Verification items for the finished model (mm, model axes). Coordinates: 2 decimals unless noted, no trailing zeros. Order: outer loops, then holes, each group sorted by start corner. A loop starts at its lowest first (then second) coordinate and runs counter-clockwise, first axis right, second up. Notation, with made-up numbers: M -21.5,-6 L -1.5,-6 A27 cw -1.5,22 Z; hole C -1.5,22 d5. An arc over 180 degrees is marked long. Return JSON: item names as keys, results as strings. Group by question number.
Q1. Section check C-C, the plane y = 13.5. Enter the section's corners in (x, z), then the cut area to 3 significant figures.
Q2. Section check B-B, the plane y = -14.5. Enter the section's corners in (x, z), then the cut area to 3 significant figures.
Q3. Go/stop test with flat-tipped pins: pin 1 Ø0.9 at (x, y) = (1, -16) entering from +Z; pin 2 Ø1.5 at (x, y) = (1.5, -24.5) entering from -Z; pin 3 Ø0.9 at (x, z) = (2, -15.5) entering from -Y. Record where each tip stops, or that it passes through.
Q4. Thickness scan on probe 1 along Y at (x, z) = (0.5, 16.5); probe 2 along Y at (x, z) = (1.6, 6.5); probe 3 along Z at (x, y) = (1.8, -13). Record the ranges inside material, lowest first.
Q5. Section check A-A, the plane z = 4. Enter the section's corners in (x, y), then the cut area to 3 significant figures.
from build123d import *

# Parameters (mm, degrees)
ESBO_O1_W                = 20
ESBO_O1_H                = 20
RESSALTO_EXTRUS_O1_DEPTH = 3


with BuildPart() as part:
    # Esboço1 → Ressalto-extrusão1 (new body)
    with BuildSketch(Plane(origin=(0, 0, 0), x_dir=(0, 0, -1), z_dir=(1, 0, 0))):
        Polygon((-18.496900578, 22.479218088), (-18.496900578, 17.479218088), (-15.496900578, 17.479218088), (-15.496900578, 12.479218088), (-18.496900578, 12.479218088), (-18.496900578, 7.479218088), (-15.496900578, 7.479218088), (-15.496900578, 2.479218088), (-18.496900578, 2.479218088), (-18.496900578, -2.520781912), (-15.496900578, -2.520781912), (-15.496900578, -7.520781912), (-18.496900578, -7.520781912), (-18.496900578, -12.520781912), (-15.496900578, -12.520781912), (-15.496900578, -17.520781912), (-18.496900578, -17.520781912), (-18.496900578, -22.520781912), (-15.496900578, -22.520781912), (-15.496900578, -27.520781912), (14.503099422, -27.520781912), (14.503099422, -22.520781912), (17.503099422, -22.520781912), (17.503099422, -17.520781912), (14.503099422, -17.520781912), (14.503099422, -12.520781912), (17.503099422, -12.520781912), (17.503099422, -7.520781912), (14.503099422, -7.520781912), (14.503099422, -2.520781912), (17.503099422, -2.520781912), (17.503099422, 2.479218088), (14.503099422, 2.479218088), (14.503099422, 7.479218088), (17.503099422, 7.479218088), (17.503099422, 12.479218088), (14.503099422, 12.479218088), (14.503099422, 17.479218088), (17.503099422, 17.479218088), (17.503099422, 22.479218088), align=None)
        with Locations((-0.496900578, -12.520781912)):
            Rectangle(ESBO_O1_W, ESBO_O1_H, mode=Mode.SUBTRACT)
    extrude(amount=RESSALTO_EXTRUS_O1_DEPTH)


solid = part.part
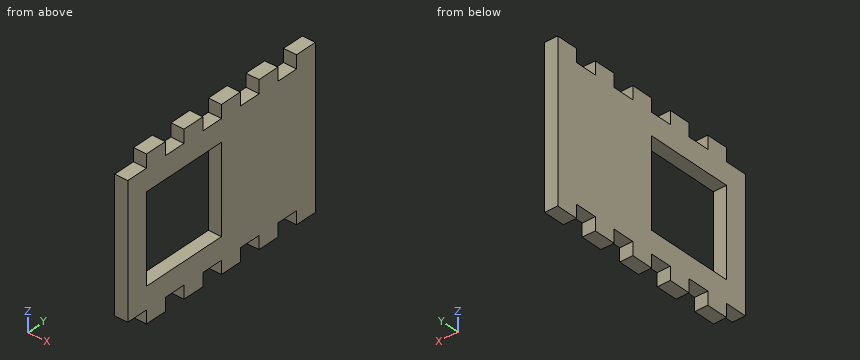
Numbers:
{
 "1": {"outline": "M 0,-14.5 L 3,-14.5 L 3,15.5 L 0,15.5 Z", "area": "90.0 mm2"},
 "2": {"outline": "M 0,-14.5 L 3,-14.5 L 3,-9.5 L 0,-9.5 Z; M 0,10.5 L 3,10.5 L 3,15.5 L 0,15.5 Z", "area": "30.0 mm2"},
 "3": {"pin 1": "stops at z = 15.5", "pin 2": "stops at z = -14.5", "pin 3": "stops at y = -22.52"},
 "4": {"probe 1": "y = -22.52 to -17.52, -12.52 to -7.52, -2.52 to 2.48, 7.48 to 12.48, 17.48 to 22.48", "probe 2": "y = -27.52 to -22.52, -2.52 to 22.48", "probe 3": "z = -14.5 to -9.5, 10.5 to 15.5"},
 "5": {"outline": "M 0,-27.52 L 3,-27.52 L 3,-22.52 L 0,-22.52 Z; M 0,-2.52 L 3,-2.52 L 3,22.48 L 0,22.48 Z", "area": "90.0 mm2"}
}
